Check sheet for the modelled part. Datum: model origin and axes. Units: mm. Give positions to 0.01 mm unless a question says otherwise; leave off trailing zeros. Loops run counter-clockwise (first coordinate to the right, second up) from the corner with the lowest first, then second, coordinate; pieces in that order, holes last.
```python
from build123d import *

# Parameters (mm, degrees)
SZKIC1_W                        = 4
SZKIC1_H                        = 25
WYTNIJ_WYCI_GNI_CIE1_DEPTH      = 13
WYTNIJ_WYCI_GNI_CIE1_DEPTH_BACK = 13
SZKIC3_R                        = 9.5
WYTNIJ_WYCI_GNI_CIE2_DEPTH      = 5
WYTNIJ_WYCI_GNI_CIE2_DEPTH_BACK = 5
SFAZOWANIE1_SIZE                = 1.25


with BuildPart() as part:
    # Szkic1 → Obrót1 (revolve)
    with BuildSketch(Plane(origin=(0, 0, 0), x_dir=(1, 0, 0), z_dir=(0, 1, 0))):
        with BuildLine():
            Line((0, 12), (0, -17))
            Line((0, -17), (4, -17))
            Line((4, -17), (10.37531088, -6.029338617))
            ThreePointArc((10.37531088, -6.029338617), (10.400770726, 5.985312715), (0, 12))
        make_face()
        with Locations((2, -29.5)):
            Rectangle(SZKIC1_W, SZKIC1_H)
    revolve(axis=Axis((0, 0, -26.043516498), (0, 0, 1)))

    # Szkic2 → Wytnij-wyciągnięcie1 (cut, two sides)
    with BuildSketch(Plane(origin=(0, 0, 0), x_dir=(0, 0, -1), z_dir=(1, 0, 0))) as wytnij_wyci_gni_cie1_sk:
        with BuildLine():
            Line((-17, 4), (11.313708499, 4))
            ThreePointArc((11.313708499, 4), (4.140324681, 11.263112871), (-6.029338617, 10.37531088))
            Line((-6.029338617, 10.37531088), (-17, 4))
        make_face()
        with BuildLine():
            Line((-17, -4), (11.313708499, -4))
            ThreePointArc((11.313708499, -4), (4.140324681, -11.263112871), (-6.029338617, -10.37531088))
            Line((-6.029338617, -10.37531088), (-17, -4))
        make_face()
    extrude(amount=WYTNIJ_WYCI_GNI_CIE1_DEPTH, mode=Mode.SUBTRACT)
    extrude(wytnij_wyci_gni_cie1_sk.sketch, amount=-WYTNIJ_WYCI_GNI_CIE1_DEPTH_BACK, mode=Mode.SUBTRACT)

    # Szkic3 → Wytnij-wyciągnięcie2 (cut, two sides)
    with BuildSketch(Plane(origin=(0, 0, 0), x_dir=(1, 0, 0), z_dir=(0, 1, 0))) as wytnij_wyci_gni_cie2_sk:
        Circle(SZKIC3_R)
    extrude(amount=WYTNIJ_WYCI_GNI_CIE2_DEPTH, mode=Mode.SUBTRACT)
    extrude(wytnij_wyci_gni_cie2_sk.sketch, amount=-WYTNIJ_WYCI_GNI_CIE2_DEPTH_BACK, mode=Mode.SUBTRACT)

    # Sfazowanie1
    sfazowanie1_edges = [part.edges().sort_by_distance(p)[0] for p in [
        (-4, 0, 42),
    ]]
    chamfer(sfazowanie1_edges, length=SFAZOWANIE1_SIZE)


solid = part.part
```
(1) Gauge pin test, flat ends, axial feed: pin 1 Ø3 at (y, z) = (2, 24) entering from +X; pin 2 Ø6 at (x, z) = (1, 29) entering from +Y; pin 3 Ø1 at (x, y) = (2.5, 3) entering from -Z; pin 4 Ø1 at (x, z) = (4.5, 14.5) entering from +Y. Record the tip position at first contact, or that the pin passes through.
(2) Section check D-D on z = 31.5. Record the boundary of the cut face in (x, y).
(3) Material ranges on line 1 (X direction, y = 1.5, z = 0); line 2 (Z direction, x = -1.5, y = -2.5); line 3 (Z direction, x = 0, y = 1.5), recorded low to high.
(4) Section check B-B on y = 0. Record the boundary of the cut face in (x, z), plus the area to 3 significant figures.
(5) Section check A-A on z = 0. Record the boundary of the cut face in (x, y).
(6) Release check for a two-part mould opening along X. For faces 1 (the face through (4.38, 0.06, 8.43)), 2 (the face through (-0.867, -3.905, 28.709)), 3 (the face through (0, 0, 42)) record: pulls with the +X half, pulls with the -X half, needs draft (parallel to the pull), parting line crosses it, or undercut.
(7) Section check C-C on z = 7.5. Record the boundary of the cut face in (x, y), plus the area to 3 significant figures.
Computed values:
1. pin 1: stops at x = 3.97
1. pin 2: stops at y = 4
1. pin 3: stops at z = -11.51
1. pin 4: stops at y = 3.85
2. outline: circle Ø8 at (0, 0)
3. line 1: x = -11.91 to -9.5, 9.5 to 11.91
3. line 2: z = -11.64 to -9.38, 9.38 to 41.83
3. line 3: z = -11.91 to -9.5, 9.5 to 42
4. outline: (-10.38, 6.03) arc R12 ccw (long way) to (10.38, 6.03) - (4, 17) - (4, 40.75) - (2.75, 42) - (-2.75, 42) - (-4, 40.75) - (-4, 17) - close; hole circle Ø19 at (0, 0)
4. area: 437 mm2
5. outline: (-11.31, -4) - (-9.5, -4) - (-9.5, 4) - (-11.31, 4) arc R12 ccw to start; (9.5, -4) - (11.31, -4) arc R12 ccw to (11.31, 4) - (9.5, 4) - close
6. face 1: undercut
6. face 2: parting line crosses it
6. face 3: needs draft
7. outline: (-8.64, -4) - (-5.83, -4) - (-5.83, 4) - (-8.64, 4) arc R9.52 ccw to start; (5.83, -4) - (8.64, -4) arc R9.52 ccw to (8.64, 4) - (5.83, 4) - close
7. area: 54.4 mm2
